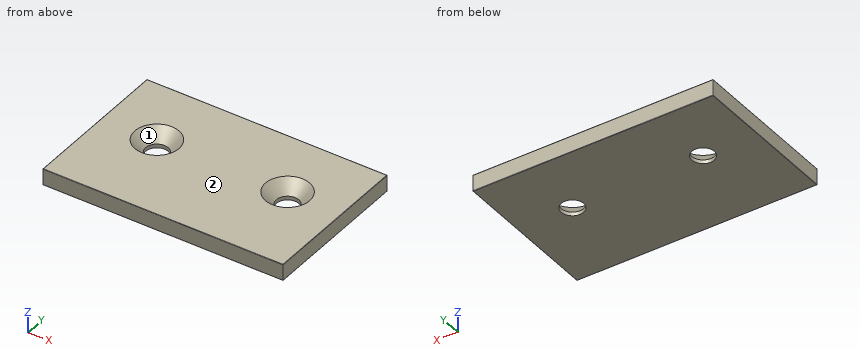
```python
from build123d import *

# Parameters (mm, degrees)
SKETCH1_W           = 69.85
SKETCH1_H           = 44.45
BOSS_EXTRUDE1_DEPTH = 2.3749
FILLET1_R           = 0.127


with BuildPart() as part:
    # Sketch1 → Boss-Extrude1 (new, symmetric)
    with BuildSketch(Plane.XY):
        with Locations((0, 22.225)):
            Rectangle(SKETCH1_W, SKETCH1_H)
    extrude(amount=BOSS_EXTRUDE1_DEPTH, both=True)

    # Sketch4 → CSK for 1/4 Flat Head Machine Screw2 (revolve, cut)
    with BuildSketch(Plane(origin=(18.998712013, 25.315105776, 2.3749), x_dir=(0, -1, 0), z_dir=(1, 0, 0))):
        Polygon((0, 0), (0, 4.7498), (3.2639, 4.7498), (3.2639, 3.652419693), (6.4389, 0), align=None)
    csk_for_1_4_flat_head_machine_screw2 = revolve(axis=Axis((18.998712013, 25.315105776, 8.7249), (0, 0, -1)), mode=Mode.SUBTRACT)

    # Mirror1: CSK for 1/4 Flat Head Machine Screw2 across plane
    add(csk_for_1_4_flat_head_machine_screw2.mirror(Plane(origin=(0, 0, 0), x_dir=(0, 0, 1), z_dir=(1, 0, 0))), mode=Mode.SUBTRACT)

    # Fillet1
    fillet1_edges = [part.edges().sort_by_distance(p)[0] for p in [
        (34.925, 22.225, 2.3749),
        (0, 44.45, 2.3749),
        (-34.925, 22.225, 2.3749),
        (0, 44.45, -2.3749),
        (34.925, 22.225, -2.3749),
        (0, 0, -2.3749),
        (-34.925, 22.225, -2.3749),
        (0, 0, 2.3749),
        (-34.925, 44.45, 0),
        (34.925, 44.45, 0),
        (34.925, 0, 0),
        (-34.925, 0, 0),
    ]]
    fillet(fillet1_edges, radius=FILLET1_R)


solid = part.part
```
For this review, take the finished solid that the model builds, in its own axes (mm). Face numbers are marked on the shaded views. Round coordinates to 2 decimals unless told otherwise and drop trailing zeros. Write each loop counter-clockwise with the first axis right and the second up, starting at its lowest first coordinate (ties: lowest second). Pieces come first, ordered by that corner, then holes. Notation, with made-up numbers: M -30,-33.75 L -11,-33.75 A15 ccw -11,-9.75 Z; hole C 56.25,-19.75 d1. An arc over 180 degrees is marked long. One line per item, written item: value. Start each with the question number.
(1) We need section B-B (y = 24). Count the separate pieces of the cut face and the enclosed holes in it, and give its area (3 significant figures).
(2) We need section A-A (z = -0.3). Give the boundary of the cut face in (x, y) (3 decimals).
(3) Wall thickness on line 1 (Y direction, x = -14.5, z = 1.5); line 2 (Y direction, x = -22.5, z = 0.25): over which ranges is each line inside the solid? List them lowest first.
(4) The part is to be moulded in two halves that separate along Y. For the marked faces 1 and 2, say which applies: released by +Y, released by -Y, zero draft, split by the parting line, or undercut.
(5) Insertion check: pin 1 (7.5 mm diameter, centred on x = -19, y = 25.32, fed in from +Z). The pin has a flat end and moves straight along its axis. Give the tip position at first contact, or say it passes through.
Result:
1. separate pieces: 3
1. enclosed holes: 0
1. area: 251 mm²
2. outline: M -34.925,0.127 A0.127 ccw -34.798,0 L 34.798,0 A0.127 ccw 34.925,0.127 L 34.925,44.323 A0.127 ccw 34.798,44.45 L -34.798,44.45 A0.127 ccw -34.925,44.323 Z; hole C -18.999,25.315 d8.227; hole C 18.999,25.315 d8.227
3. line 1: 0 to 21.85, 28.78 to 44.45
3. line 2: 0 to 22.34, 28.29 to 44.45
4. face 1: undercut
4. face 2: zero draft
5. pin 1: z = -0.71
